Build history of the part. All positions in model axes, mm. Give positions to 0.01 mm unless a question says otherwise; leave off trailing zeros. Loops run counter-clockwise (first coordinate to the right, second up) from the corner with the lowest first, then second, coordinate; pieces in that order, holes last. Notation, with made-up numbers: M 54.25,61 L 102.25,61 A10 cw 102.25,69 Z; hole C 22,19 d9. An arc over 180 degrees is marked long. Answer in a Markdown table with one row per item. Add a question column.
```python
from build123d import *

# Parameters (mm, degrees)
SKETCH1_R           = 1.5
SKETCH1_R_2         = 3.45
BOSS_EXTRUDE1_DEPTH = 1.5


with BuildPart() as part:
    # Sketch1 → Boss-Extrude1 (new body, symmetric)
    with BuildSketch(Plane(origin=(0, 0, 0), x_dir=(1, 0, 0), z_dir=(0, 1, 0))):
        with BuildLine():
            Line((19.451315789, 3.470780036), (0.767236842, 5.900326061))
            ThreePointArc((0.767236842, 5.900326061), (-5.95, 0), (0.767236842, -5.900326061))
            Line((0.767236842, -5.900326061), (19.451315789, -3.470780036))
            ThreePointArc((19.451315789, -3.470780036), (22.5, 0), (19.451315789, 3.470780036))
        make_face()
        with Locations((19, 0)):
            Circle(SKETCH1_R, mode=Mode.SUBTRACT)
        Circle(SKETCH1_R_2, mode=Mode.SUBTRACT)
    extrude(amount=BOSS_EXTRUDE1_DEPTH, both=True)


solid = part.part
```
(1) Wall check: line 1 (X direction, y = 0.55, z = 0); line 2 (Z direction, x = 0, y = -0.2); line 3 (X direction, y = -1.2, z = 0.75). Give the ranges that are in metal, low to high.
(2) Pull direction X, two halves, no side cores. Call faces 1 (the flat face through (8, 1.5, 0)), 2 (the cylindrical face through (22.5, 0, 0.1)), 3 (the cylindrical face through (17.5, -0.02, -0.07)): +X half, -X half, draft (parallel to the pull), parting line (faces both ways), or undercut.
(3) Slice it at A-A, the plane x = 0. Give the cut face in (y, z), then the cut area to 3 significant figures.
(4) Slice it at C-C, the plane y = 1. Give the cut face in (x, z).
(5) Slice it at B-B, the plane z = 0. Give the cut face in (x, y).
(6) Pin check, flat tip, straight feed: pin 1 (1.5 mm diameter, centred on y = 0, z = -2, fed in from +X). Stop position of the tip, or through.
(7) Slice it at D-D, the plane z = 2. Give the cut face in (x, y), then the cut area to 3 significant figures.
Solution:
| question | item | result |
|---|---|---|
| 1 | line 1 | -5.95 to -3.45, 3.45 to 17.5, 20.5 to 22.5 |
| 1 | line 2 | -5.95 to -3.45, 3.45 to 5.95 |
| 1 | line 3 | -5.9 to -3.37, 3.37 to 17.7, 20.3 to 22.42 |
| 2 | face 1 | draft |
| 2 | face 2 | +X half |
| 2 | face 3 | undercut |
| 3 | outline | M -1.5,-5.95 L 1.5,-5.95 L 1.5,-3.45 L -1.5,-3.45 Z; M -1.5,3.45 L 1.5,3.45 L 1.5,5.95 L -1.5,5.95 Z |
| 3 | area | 15.0 mm^2 |
| 4 | outline | M 0.77,-5.9 L 19.45,-3.47 A3.5 ccw 19.45,3.47 L 0.77,5.9 A5.95 ccw long Z; hole C 0,0 d6.9; hole C 19,0 d3 |
| 5 | outline | M -5.95,-1.5 L -3.45,-1.5 L -3.45,1.5 L -5.95,1.5 Z; M 3.45,-1.5 L 17.5,-1.5 L 17.5,1.5 L 3.45,1.5 Z; M 20.5,-1.5 L 22.5,-1.5 L 22.5,1.5 L 20.5,1.5 Z |
| 6 | pin 1 | x = 22.27 |
| 7 | outline | M -5.6,-1.5 L -2.81,-1.5 L -2.81,1.5 L -5.6,1.5 Z; M 2.81,-1.5 L 21.87,-1.5 L 21.87,1.5 L 2.81,1.5 Z |
| 7 | area | 65.6 mm^2 |
